The model under review builds one solid part; all positions refer to its coordinate system, in mm. A direction names the side the tool comes from. Give positions to 0.01 mm unless a question says otherwise; leave off trailing zeros. Order: outer loops, then holes, each group sorted by start corner. A loop starts at its lowest first (then second) coordinate and runs counter-clockwise, first axis right, second up. Notation, with made-up numbers: (68, 83) - (75, 83) arc R18 ccw to (75, 95) - close; hole circle Ø11 at (-40, 70). An arc over 180 degrees is marked (long way). Use a Markdown table: item, result. Add a question column.
```python
from build123d import *

# Parameters (mm, degrees)
SKETCH2_R           = 1.15
BOSS_EXTRUDE1_DEPTH = 2
SKETCH3_R           = 1.5
BOSS_EXTRUDE2_DEPTH = 5
FILLET1_R           = 5


with BuildPart() as part:
    # Sketch2 → Boss-Extrude1 (new body)
    with BuildSketch(Plane(origin=(0, 0, 0), x_dir=(1, 0, 0), z_dir=(0, 1, 0))):
        with BuildLine():
            Line((4.000381204, 4.673041052), (12.000381204, 5.468452872))
            Line((12.000381204, 5.468452872), (13.182938655, 15.86470146))
            ThreePointArc((13.182938655, 15.86470146), (12.256191848, 17.552341108), (10.334811071, 17.675966101))
            Line((10.334811071, 17.675966101), (3.154801126, 14.147870696))
            ThreePointArc((3.154801126, 14.147870696), (3.968738574, 9.44536378), (4.000381204, 4.673041052))
        make_face()
        with Locations(Location((11.182938655, 15.86470146, 0), (0, 0, 270))):
            Circle(SKETCH2_R, mode=Mode.SUBTRACT)
    extrude(amount=BOSS_EXTRUDE1_DEPTH)

    # Sketch3 → Boss-Extrude2 (add)
    with BuildSketch(Plane(origin=(0, 0, 0), x_dir=(1, 0, 0), z_dir=(0, 1, 0))):
        with Locations(Location((10.487550657, 9.86470146, 0), (0, 0, 270))):
            Circle(SKETCH3_R)
    extrude(amount=-BOSS_EXTRUDE2_DEPTH)

    # Fillet1
    fillet1_edges = [part.edges().sort_by_distance(p)[0] for p in [
        (3.154801126, 1, -14.147870696),
    ]]
    fillet(fillet1_edges, radius=FILLET1_R)


solid = part.part
```
Q1. We need section C-C (x = 7.75). Write out the cut boundary in (y, z).
Q2. We need section D-D (y = -4). Write out the cut boundary in (x, z).
Q3. Machinability: for faces 1 (the cylindrical face through (9.023, -2.465, -10.19)), 2 (the cylindrical face through (4.07, 0.99, -7.73)), which of the approach directions +Z, -Z, +X, -X, +Y, -Y give a long, thin tool a straight path to every point of the face, cutting with its end or side? Answer none if there is none.
Q4. Clearance check with flat-ended pins moving along their axes: P1, Ø4, axis at x = 8.5, y = 1, coming from the +Z side; P2, Ø4, axis at x = 8, y = -3.5, coming from the +Z side; P3, Ø3, axis at x = 7, z = -12, coming from the -Y side. State where each tip first meets the part, or that it passes through.
Q5. Wall thickness on probe 1 along Y at (x, z) = (8.75, -15.5); probe 2 along Z at (x, y) = (10.75, 1); probe 3 along X at (y, z) = (-1.5, -9.75): over which ranges is each line inside the solid? List them lowest first.
Q6. We need section B-B (z = -9). Write out the cut boundary in (x, y).
Q7. We need section A-A (z = -15.5). Write out the cut boundary in (x, y).
Q8. Draft analysis for pull direction X (two halves, no side actions). For faces 3 (the flat face through (12.583, 0.986, -10.594)), 4 (the cylindrical face through (11.53, 0.99, -14.77)), 5 (the flat face through (8.485, 0.986, -16.767)), state which applies: pulls with the +X half, pulls with the -X half, needs draft (parallel to the pull), parting line crosses it, or undercut.
Here are the results:
| question | item | result |
|---|---|---|
| 1 | outline | (0, -16.41) - (2, -16.41) - (2, -5.05) - (0, -5.05) - close |
| 2 | outline | circle Ø3 at (10.49, -9.86) |
| 3 | face 1 | -Y |
| 3 | face 2 | -X, +Y, -Y |
| 4 | P1 | z = -4.92 |
| 4 | P2 | z = -8.45 |
| 4 | P3 | y = 0 |
| 5 | probe 1 | 0 to 2 |
| 5 | probe 2 | -17.82 to -16.93, -14.8 to -5.34 |
| 5 | probe 3 | 8.99 to 11.98 |
| 6 | outline | (4.01, 0) - (9.26, 0) - (9.26, -5) - (11.71, -5) - (11.71, 0) - (12.4, 0) - (12.4, 2) - (4.01, 2) - close |
| 7 | outline | (6.01, 0) - (10.09, 0) - (10.09, 2) - (6.01, 2) - close; (12.27, 0) - (13.14, 0) - (13.14, 2) - (12.27, 2) - close |
| 8 | face 3 | pulls with the +X half |
| 8 | face 4 | undercut |
| 8 | face 5 | pulls with the -X half |
